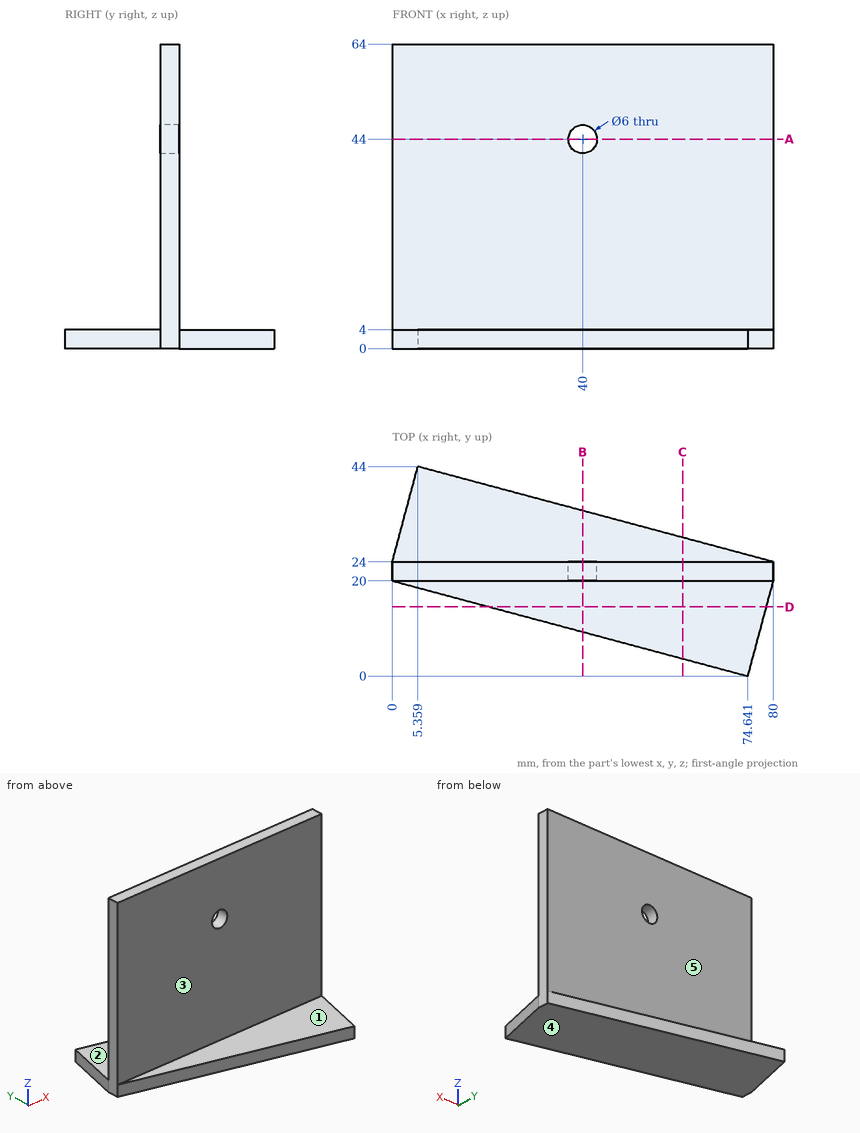
Source: three-view drawing plus pictorial views. Frame: mm from the lowest corner of the part. A direction names the side the tool comes from. Round coordinates to 2 decimals unless told otherwise and drop trailing zeros. Loops run counter-clockwise (first coordinate to the right, second up) from the corner with the lowest first, then second, coordinate; pieces in that order, holes last.
Item 1: Section C-C, the plane x = 61. Output: boundary loops of the cut face in (y, z).
Checked values:
outline: (3.66, 0) - (29.09, 0) - (29.09, 4) - (24, 4) - (24, 64) - (20, 64) - (20, 4) - (3.66, 4) - close
Item 2: Section A-A, the plane z = 44. Output: boundary loops of the cut face in (x, y), plus the area to 3 significant figures.
Checked values:
outline: (0, 20) - (37, 20) - (37, 24) - (0, 24) - close; (43, 20) - (80, 20) - (80, 24) - (43, 24) - close
area: 296 mm2
Item 3: Mould query, pull axis Y, two halves, no side actions, for the marked faces 3, 4 and 5. Classes: released by +Y, released by -Y, zero draft, split by the parting line, or undercut.
Checked values:
face 3: released by -Y
face 4: zero draft
face 5: released by +Y
Item 4: Contact query for flat-ended pins moving along their axis: P1, Ø12, axis at x = 22.5, z = 56.5, coming from the -Y side; P2, Ø1.5, axis at x = 30.5, z = 31, coming from the +Y side; P3, Ø1.5, axis at x = 8, y = 26.5, coming from the +Z side. Output: stop coordinate, or through.
Checked values:
P1: stops at y = 20
P2: stops at y = 24
P3: stops at z = 4
Item 5: Section D-D, the plane y = 14.5. Output: boundary loops of the cut face in (x, z).
Checked values:
outline: (20.53, 0) - (78.53, 0) - (78.53, 4) - (20.53, 4) - close
Item 6: Line query: L1, parallel to X at y = 22.6, z = 44; L2, parallel to Y at x = 21, z = 8; L3, parallel to Z at x = 52, y = 10.5. Output: solid intervals per line, ascending.
Checked values:
L1: x = 0 to 37, 43 to 80
L2: y = 20 to 24
L3: z = 0 to 4
Item 7: Reachability of the marked faces 1 and 2 from +Z, -Z, +X, -X, +Y, -Y: full face, straight path, thin tool, end or side. Return the list, or none.
Checked values:
face 1: +Z, +X, -X, -Y
face 2: +Z, +X, -X, +Y
Item 8: Section B-B, the plane x = 40. Output: boundary loops of the cut face in (y, z).
Checked values:
outline: (9.28, 0) - (34.72, 0) - (34.72, 4) - (24, 4) - (24, 41) - (20, 41) - (20, 4) - (9.28, 4) - close; (20, 47) - (24, 47) - (24, 64) - (20, 64) - close
